CAD build for the part. Positions are in the model's coordinates, mm. A direction names the side the tool comes from. Give positions to 0.01 mm unless a question says otherwise; leave off trailing zeros. Loops run counter-clockwise (first coordinate to the right, second up) from the corner with the lowest first, then second, coordinate; pieces in that order, holes last. Notation, with made-up numbers: (50, -34) -> (107, -34) arc R37 ccw to (107, 3) -> close; hole circle Ø4 at (-11, 77.5). An arc over 180 degrees is marked (long way). Use one line per item in the form item = value.
```python
from build123d import *

# Parameters (mm, degrees)
SKETCH1_R           = 4.75
BOSS_EXTRUDE1_DEPTH = 10
BOSS_EXTRUDE1_DRAFT = -4
SKETCH2_R           = 2.75
CUT_EXTRUDE1_DEPTH  = 4
FILLET1_R           = 1


with BuildPart() as part:
    # Sketch1 → Boss-Extrude1 (with draft: the straight prism first)
    with BuildSketch(Plane(origin=(0, 0, 0), x_dir=(1, 0, 0), z_dir=(0, 1, 0))):
        Circle(SKETCH1_R)
    extrude(amount=-BOSS_EXTRUDE1_DEPTH)
    # Boss-Extrude1: the draft: its side faces are tilted about the plane it starts from
    boss_extrude1_sides = [part.faces().sort_by_distance(p)[0] for p in [
        (-4.75, -5, 0),
    ]]
    draft(boss_extrude1_sides, Plane(origin=(0, 0, 0), x_dir=(1, 0, 0), z_dir=(0, 1, 0)), BOSS_EXTRUDE1_DRAFT)

    # Sketch2 → Cut-Extrude1 (cut)
    with BuildSketch(Plane(origin=(0, 0, 0), x_dir=(1, 0, 0), z_dir=(0, 1, 0))):
        with Locations(Location((0, 0, 0), (0, 0, 270))):
            Circle(SKETCH2_R)
    extrude(amount=-CUT_EXTRUDE1_DEPTH, mode=Mode.SUBTRACT)

    # Fillet1
    fillet1_edges = [part.edges().sort_by_distance(p)[0] for p in [
        (-4.050731881, -10, 0),
    ]]
    fillet(fillet1_edges, radius=FILLET1_R)


solid = part.part
```
1. Drill centre lines: line 1 (Y direction, x = -1, z = 1.5); line 2 (X direction, y = -1, z = -2.25); line 3 (X direction, y = -1.7, z = 0). Where is each one in solid material? Low to high.
Result sheet:
line_1 = -10 to -4
line_2 = -4.1 to -1.58, 1.58 to 4.1
line_3 = -4.63 to -2.75, 2.75 to 4.63
2. Cut at C-C, the plane y = -5.5. Write the cut outline in (x, z), then the cut area to 3 significant figures.
Result sheet:
outline = circle Ø8.73 at (0, 0)
area = 59.9 mm^2
3. Drop flat-ended pins along their axis: P1, Ø2, axis at y = -5, z = 0, coming from the +X side; P2, Ø4.5, axis at x = 0, z = 0, coming from the +Y side; P3, Ø1.5, axis at x = 3, z = 3, coming from the -Y side. Give the stop position or say it passes through.
Result sheet:
P1 = 4.47
P2 = -4
P3 = -9.93
4. Tool access for faces 1 (the flat face through (0, -10, 0)), 2 (the cylindrical face through (-2.685, -1.972, -0.596)): list every direction of +Z, -Z, +X, -X, +Y, -Y with a clear straight run to the whole face (end or side of a thin tool).
Result sheet:
face_1 = +Z, -Z, +X, -X, -Y
face_2 = +Y
5. Mould opens along X. For faces 3 (the flat face through (0, -4, 0)), 4 (the conical face through (-0.962, -4.471, 4.332)), 5 (the flat face through (0, 0, 3)) say: pulls with the +X half, pulls with the -X half, needs draft (parallel to the pull), parting line crosses it, or undercut.
Result sheet:
face_3 = undercut
face_4 = parting line crosses it
face_5 = needs draft
6. Cut at A-A, the plane x = 0. Write the cut outline in (y, z).
Result sheet:
outline = (-10, -3.12) arc R1 ccw to (-9.07, -4.12) -> (0, -4.75) -> (0, -2.75) -> (-4, -2.75) -> (-4, 2.75) -> (0, 2.75) -> (0, 4.75) -> (-9.07, 4.12) arc R1 ccw to (-10, 3.12) -> close
7. Cut at B-B, the plane y = -1. Write the cut outline in (x, z).
Result sheet:
outline = circle Ø9.36 at (0, 0); hole circle Ø5.5 at (0, 0)
